Geometry: final body of the model. Coordinates: model frame, mm. A direction names the side the tool comes from. Round coordinates to 2 decimals unless told otherwise and drop trailing zeros. Order: outer loops, then holes, each group sorted by start corner. A loop starts at its lowest first (then second) coordinate and runs counter-clockwise, first axis right, second up. Notation, with made-up numbers: (-7, 40.5) - (42, 40.5) arc R21 ccw to (42, 44.5) - close; hole circle Ø11 at (-21.5, 58.5). An arc over 180 degrees is marked (long way). Put each result on its own line as item: value. Start each with the question number.
(1) Pin query (flat end, axial travel): P1, Ø6, axis at x = 9.5, y = -1.5, coming from the +Z side; P2, Ø1, axis at x = 47.5, z = 4, coming from the -Y side; P3, Ø6, axis at x = 87, y = -3.5, coming from the -Z side. Return the tip coordinate at first contact, or that it passes through.
(2) Access query for faces 1 (the face through (-0.4, 7, 0)), 2 (the face through (-5.5, 0, 0)), 3 (the face through (-0.4, -7, 0)), 4 (the face through (0, 3, -3)). Directions: +Z, -Z, +X, -X, +Y, -Y. A direction counts if a zero-diameter tool reaches every point of the face in a straight line with its end or side. Return the directions, or none.
(3) Section A-A (x = 20). Output: boundary loops of the cut face in (y, z), and give its area (3 significant figures).
(4) Material intervals for L1, parallel to X at y = 4.5, z = -2; L2, parallel to Z at x = 56, y = 3.5; L3, parallel to Y at x = 27.5, z = 3, sorted ascending. Write a range as [from, to].
Autodesk Inventor part; units mm, degrees
ref_plane "Work Plane1" through (1.525, 0, 0) normal (0, 0, 1) x (1, 0, 0)
ref_plane "YZ Plane" through (0, 0, 0) normal (1, 0, 0) x (0, 1, 0)
ref_plane "XZ Plane" through (0, 0, 0) normal (0, 1, 0) x (-1, 0, 0)
sketch "Sketch1" plane through (0, 0, 0) normal (0, 0, 1) x (1, 0, 0)
  line L0 (0, 6.5) -> (0, 4)
  line L1 (78, 4) -> (100, 4)
  line L2 (100, 4) -> (100, 0)
  line L3 (100, 0) -> (-0.4001, 0)
  line L4 (-20.4801, 0) -> (120.08, 0)
  line L5 (-0.4001, 0) -> (-0.4001, 6.5)
  line L6 (-0.4001, 6.5) -> (0, 6.5)
  line L7 (78, 4) -> (77.3864, 4)
  line L8 (77.3864, 4) -> (0, 4)
  line L9 (0, -1.3) -> (0, 7.8)
  dimension "d0" = 100
  dimension "d1" = 22
  dimension "d2" = 8
  dimension "d9" = 0.4001
  dimension "d10" = 13
  dimension "d13" = 0.6136
  dimension "d14" = 8
revolve "Body" add sketch "Sketch1" angle 360 about axis through (100, 0, 0) along (-1, 0, 0)
sketch "Sketch2" plane through (-0.4001, 0, 0) normal (-1, 0, 0) x (0, 0, 1)
  line L0 (0, 7.5056) -> (6.5, 3.7528)
  line L1 (6.5, 3.7528) -> (6.5, -3.7528)
  line L2 (6.5, -3.7528) -> (0, -7.5056)
  line L3 (0, -7.5056) -> (-6.5, -3.7528)
  line L4 (-6.5, -3.7528) -> (-6.5, 3.7528)
  line L5 (-6.5, 3.7528) -> (0, 7.5056)
  point P0 (0, 0)
  point P1 (0, 0)
  dimension "d11" = 13
extrude "Head" add sketch "Sketch2" along normal blind 5.1
sketch "Sketch4" plane through (0, 0, 0) normal (0, 0, 1) x (1, 0, 0)
  line L0 (-5.5001, 6.5) -> (-5.5001, 7.5056)
  line L1 (-5.5001, 7.5056) -> (-4.9195, 7.5056)
  line L2 (-4.9195, 7.5056) -> (-5.5001, 6.5)
  line L3 (-6.5201, 0) -> (0.6199, 0)
  line L4 (-0.4001, 7.5056) -> (-5.5001, 7.5056)
  line L5 (-5.5001, 3.7528) -> (-5.5001, 7.5056)
  dimension "d5" = 30
  dimension "d19" = 13
revolve "Chamfer1" cut sketch "Sketch4" angle 360 about axis through (-10, 0, 0) along (1, 0, 0)
thread "Thread"
chamfer "Chamfer2" distance 0.6134 distance2 0.6136 1 edges at (100, -4, 0) measured on face at (100, -1.054, 1.6624)
ref_plane "Work Plane1" through (1.525, 0, 0) normal (0, 0, 1) x (1, 0, 0)
equation "\"d0\" = NLG"
equation "\"d1\" = GEL"
equation "\"d2\" = GD"
equation "\"d10\" = SD2"
equation "\"d14\" = BDM"
equation "\"d11\" = SW"
equation "\"d3\" = KOH - SD"
equation "\"d5\" = ANG1"
equation "\"d19\" = SW0"
equation "\"d15\" = GEL"
equation "\"d6\" = -0.5 * SPD + 0.5 * GD"
equation "\"NLG\" = 100"
equation "\"GD\" = NND"
equation "\"BDM\" = NND"
equation "\"KOH\" = 5.5"
equation "\"GEL\" = 22"
equation "\"SW\" = 13"
equation "\"SW0\" = SW"
equation "\"SPD\" = NND - 1.2269 * PTC"
equation "\"SD2\" = SW"
equation "\"SD\" = WFT"
equation "\"ANG1\" = 30deg"
equation "\"GAL\" = 0.61345 * PTC"
equation "\"GUL\" = 0.61345 * PTC"
equation "\"RR\" = 0.4"
equation "\"WFT\" = 0.4"
equation "\"GD1\" = THREADDIA - 1.2269 * PTC"
equation "\"THREADDIA\" = 8"
equation "\"SDH\" = SW"
equation "\"TOA\" = 30deg"
equation "\"PTC\" = 1"
equation "\"NND\" = 8"
equation "\"E0\" = 1.155 * SW"
properties part number "CNS 4320 - M8 x 100" material "Steel, Mild"
Checks:
1. P1: stops at z = 4
1. P2: stops at y = -1.94
1. P3: stops at z = -3.97
2. face 1: +X, +Y
2. face 2: +Z, -Z, -X, +Y, -Y
2. face 3: +X, -Y
2. face 4: +X
3. outline: circle Ø8 at (0, 0)
3. area: 50.3 mm²
4. L1: x = [-5.5, 0]
4. L2: z = [-1.94, 1.94]
4. L3: y = [-2.65, 2.65]
